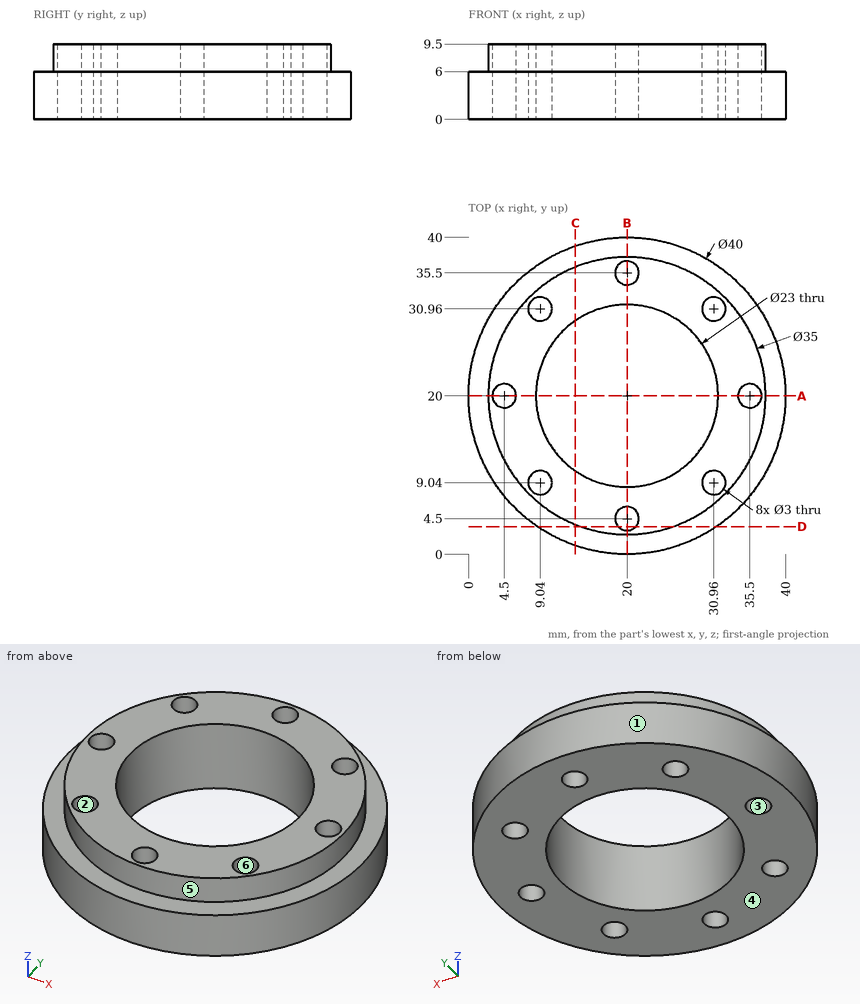
Source: three-view drawing plus pictorial views. Frame: mm from the lowest corner of the part. A direction names the side the tool comes from. Give positions to 0.01 mm unless a question says otherwise; leave off trailing zeros. Write each loop counter-clockwise with the first axis right and the second up, starting at its lowest first coordinate (ties: lowest second). Pieces come first, ordered by that corner, then holes. Notation, with made-up numbers: (59, -1) - (106, -1) arc R26 ccw to (106, 38) - close; hole circle Ø11 at (5, -4.75). An arc over 180 degrees is marked (long way). Write item = value, one per line. Start each with the question number.
1. Access query for the marked faces 5 and 6. Directions: +Z, -Z, +X, -X, +Y, -Y. A direction counts if a zero-diameter tool reaches every point of the face in a straight line with its end or side. Return the directions, or none.
2. Ray query, L1, parallel to Y at x = 20, z = 5.5; L2, parallel to Y at x = 20, z = 6.25; L3, parallel to X at y = 11, z = 6.75. Return the intervals inside material, ascending.
3. Section query D-D, the plane y = 3.5. Output: boundary loops of the cut face in (x, z), then the cut area to 3 significant figures.
4. First-contact query: pin 1 Ø8 at (x, y) = (10.5, 4) entering from +Z; pin 2 Ø4 at (x, y) = (14, 14) entering from +Z; pin 3 Ø2 at (x, z) = (19.5, 3) entering from -Y; pin 4 Ø3 at (x, z) = (10.5, 4) entering from -Y. Flat tips, straight axial feed; report the tip coordinate or a pass-through.
5. Section query C-C, the plane x = 13.5. Output: boundary loops of the cut face in (y, z), then the cut area to 3 significant figures.
6. Mould query, pull axis X, two halves, no side actions, for the marked faces 1, 2, 3 and 4. Classes: released by +X, released by -X, zero draft, split by the parting line, or undercut.
7. Section query A-A, the plane y = 20. Output: boundary loops of the cut face in (x, z), then the cut area to 3 significant figures.
Check sheet entries:
q1.face_5 = +Z
q1.face_6 = +Z, -Z
q2.L1 = 0 to 3, 6 to 8.5, 31.5 to 34, 37 to 40
q2.L2 = 2.5 to 3, 6 to 8.5, 31.5 to 34, 37 to 37.5
q2.L3 = 4.99 to 12.84, 27.16 to 35.01
q3.outline = (8.7, 0) - (18.88, 0) - (18.88, 9.5) - (14.17, 9.5) - (14.17, 6) - (8.7, 6) - close; (21.12, 0) - (31.3, 0) - (31.3, 6) - (25.83, 6) - (25.83, 9.5) - (21.12, 9.5) - close
q3.area = 155 mm2
q4.pin_1 = 9.5
q4.pin_2 = through
q4.pin_3 = 0
q4.pin_4 = 1.67
q5.outline = (1.09, 0) - (10.51, 0) - (10.51, 9.5) - (3.75, 9.5) - (3.75, 6) - (1.09, 6) - close; (29.49, 0) - (38.91, 0) - (38.91, 6) - (36.25, 6) - (36.25, 9.5) - (29.49, 9.5) - close
q5.area = 160 mm2
q6.face_1 = split by the parting line
q6.face_2 = undercut
q6.face_3 = undercut
q6.face_4 = zero draft
q7.outline = (0, 0) - (3, 0) - (3, 9.5) - (2.5, 9.5) - (2.5, 6) - (0, 6) - close; (6, 0) - (8.5, 0) - (8.5, 9.5) - (6, 9.5) - close; (31.5, 0) - (34, 0) - (34, 9.5) - (31.5, 9.5) - close; (37, 0) - (40, 0) - (40, 6) - (37.5, 6) - (37.5, 9.5) - (37, 9.5) - close
q7.area = 87.0 mm2
